Input: part model. Units: mm. Frame: model coordinates. Round coordinates to 2 decimals unless told otherwise and drop trailing zeros. Loops run counter-clockwise (first coordinate to the right, second up) from the corner with the lowest first, then second, coordinate; pieces in that order, holes last. Notation, with made-up numbers: (45, -30.5) - (100, -30.5) arc R29 ccw to (100, 0.5) - close; hole circle Ø9 at (6, 40). An arc over 180 degrees is marked (long way). Write each question's results on one line, items separated by ' | '.
from build123d import *

# Parameters (mm, degrees)
SKETCH_1_W          = 70
SKETCH_1_H          = 4
EXTRUDE_1_DEPTH     = 39
SKETCH_2_R          = 13
SKETCH_2_R_2        = 3
CUT_EXTRUDE_1_DEPTH = 5


with BuildPart() as part:
    # 草图1 → 凸台-拉伸1 (new body)
    with BuildSketch(Plane.XY):
        with Locations((35, -2)):
            Rectangle(SKETCH_1_W, SKETCH_1_H)
    extrude(amount=EXTRUDE_1_DEPTH)

    # 草图2 → 切除-拉伸1 (cut)
    with BuildSketch(Plane(origin=(0, 0, 0), x_dir=(1, 0, 0), z_dir=(0, 1, 0))):
        with Locations(Location((35, -19.5, 0), (0, 0, 270))):
            Circle(SKETCH_2_R)
        with Locations(Location((7.5, -7, 0), (0, 0, 270))):
            Circle(SKETCH_2_R_2)
        with Locations(Location((62.5, -7, 0), (0, 0, 270))):
            Circle(SKETCH_2_R_2)
        with Locations(Location((62.5, -32, 0), (0, 0, 270))):
            Circle(SKETCH_2_R_2)
        with Locations(Location((7.5, -32, 0), (0, 0, 270))):
            Circle(SKETCH_2_R_2)
    extrude(amount=-CUT_EXTRUDE_1_DEPTH, mode=Mode.SUBTRACT)


solid = part.part
1. Mould query, pull axis Z, two halves, no side actions, for faces 1 (the flat face through (35, -2, 39)), 2 (the cylindrical face through (62.6, -2, 29)), 3 (the flat face through (70, -2, 19)). Classes: pulls with the +Z half, pulls with the -Z half, needs draft (parallel to the pull), parting line crosses it, or undercut.
Answer:
face 1: pulls with the +Z half | face 2: undercut | face 3: needs draft
2. Section query D-D, the plane z = 8. Output: boundary loops of the cut face in (x, y).
Answer:
outline: (0, -4) - (4.67, -4) - (4.67, 0) - (0, 0) - close; (10.33, -4) - (28.94, -4) - (28.94, 0) - (10.33, 0) - close; (41.06, -4) - (59.67, -4) - (59.67, 0) - (41.06, 0) - close; (65.33, -4) - (70, -4) - (70, 0) - (65.33, 0) - close
3. Section query A-A, the plane z = 19.5. Output: boundary loops of the cut face in (x, y), plus the area to 3 significant figures.
Answer:
outline: (0, -4) - (22, -4) - (22, 0) - (0, 0) - close; (48, -4) - (70, -4) - (70, 0) - (48, 0) - close | area: 176 mm^2
4. Section query C-C, the plane x = 62.5. Output: boundary loops of the cut face in (y, z), plus the area to 3 significant figures.
Answer:
outline: (-4, 0) - (0, 0) - (0, 4) - (-4, 4) - close; (-4, 10) - (0, 10) - (0, 29) - (-4, 29) - close; (-4, 35) - (0, 35) - (0, 39) - (-4, 39) - close | area: 108 mm^2
5. Section query B-B, the plane y = -1.7. Output: boundary loops of the cut face in (x, z).
Answer:
outline: (0, 0) - (70, 0) - (70, 39) - (0, 39) - close; hole circle Ø6 at (7.5, 7); hole circle Ø6 at (7.5, 32); hole circle Ø26 at (35, 19.5); hole circle Ø6 at (62.5, 7); hole circle Ø6 at (62.5, 32)
6. Line query: line 1 (X direction, y = -2.2, z = 19.5); line 2 (X direction, y = -0.2, z = 5); line 3 (Z direction, x = 35.5, y = -2.5). Output: solid intervals per line, ascending. Write a range as [from, to].
Answer:
line 1: [0, 22], [48, 70] | line 2: [0, 5.26], [9.74, 60.26], [64.74, 70] | line 3: [0, 6.51], [32.49, 39]
